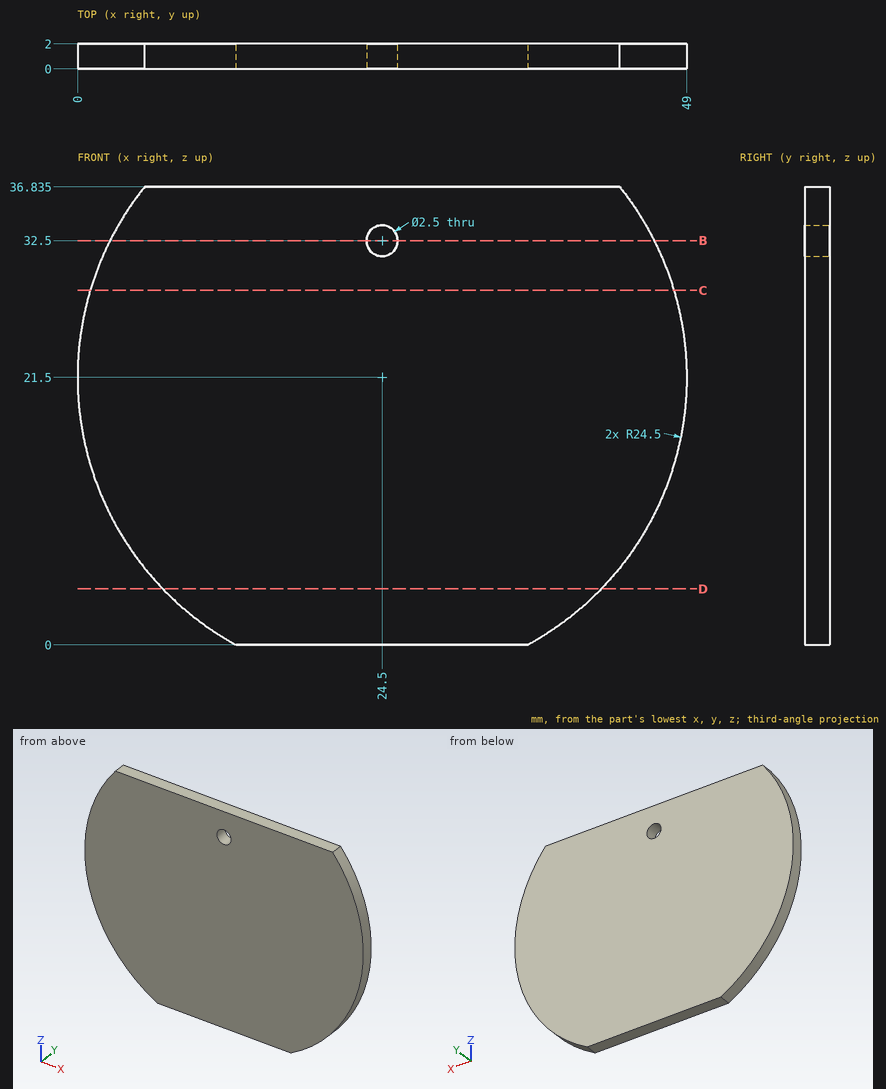
Study the drawing (mm; zero at the part's minimum x, y, z) and answer. Coordinates: 2 decimals unless noted, no trailing zeros. Loops run counter-clockwise (first coordinate to the right, second up) from the corner with the lowest first, then second, coordinate; pieces in that order, holes last. Notation, with made-up numbers: (13.5, 61) -> (51.5, 61) arc R28 ccw to (51.5, 97) -> close; hole circle Ø4 at (59, 46.25). An arc over 180 degrees is marked (long way). Answer in a Markdown table with one row per item. Add a question column.
1. Consider line 1 (X direction, y = 0.5, z = 32.5); line 2 (X direction, y = 1.9, z = 21.5); line 3 (Z direction, x = 12, y = 0.75) (1 decimal). Determine where each line is inside the solid, lowest interval first. Write a range as [from, to].
2. The part is cut by section C-C, the plane z = 28.5. Write down the section's boundary in (x, y).
3. The part is cut by section D-D, the plane z = 4.5. Write down the section's boundary in (x, y).
4. The part is cut by section B-B, the plane z = 32.5. Write down the section's boundary in (x, y), then the cut area to 3 significant figures.
5. A flat-ended cylindrical pin translates along its axis: P1, Ø1, axis at y = 1, z = 11.5, coming from the -X side. Find the tip coordinate at first contact, or state that the pin passes through.
Answer below:
| question | item | result |
|---|---|---|
| 1 | line 1 | [2.61, 23.25], [25.75, 46.39] |
| 1 | line 2 | [0, 49] |
| 1 | line 3 | [0.4, 36.8] |
| 2 | outline | (1.02, 0) -> (47.98, 0) -> (47.98, 2) -> (1.02, 2) -> close |
| 3 | outline | (6.86, 0) -> (42.14, 0) -> (42.14, 2) -> (6.86, 2) -> close |
| 4 | outline | (2.61, 0) -> (23.25, 0) -> (23.25, 2) -> (2.61, 2) -> close; (25.75, 0) -> (46.39, 0) -> (46.39, 2) -> (25.75, 2) -> close |
| 4 | area | 82.6 mm2 |
| 5 | P1 | x = 1.92 |
